Can you work these out from the model? Positions are in its coordinate system, mm. A direction names the side the tool comes from. Give positions to 0.01 mm unless a question says otherwise; leave off trailing zeros. Write each loop counter-clockwise with the first axis right and the second up, starting at its lowest first coordinate (ties: lowest second). Pieces come first, ordered by that corner, then holes.
Autodesk Inventor part; units mm, degrees
ref_plane "YZ Plane" through (0, 0, 0) normal (1, 0, 0) x (0, 1, 0)
ref_plane "XZ Plane" through (0, 0, 0) normal (0, 1, 0) x (-1, 0, 0)
ref_plane "XY Plane" through (0, 0, 0) normal (0, 0, 1) x (1, 0, 0)
sketch "Sketch1" plane through (0, 0, 0) normal (0, 0, 1) x (1, 0, 0)
  line L0 (5, 0) -> (95, 0)
  line L1 (100, 5) -> (100, 26.714)
  line L2 (95, 31.714) -> (5, 31.714)
  line L3 (0, 26.714) -> (0, 5)
  arc A0 (5, 31.714) -> (0, 26.714) centre (5, 26.714) ccw
  arc A1 (0, 5) -> (5, 0) centre (5, 5) ccw
  circle A2 centre (5, 5) radius 2.75
  circle A3 centre (5, 26.714) radius 2.75
  circle A4 centre (25, 26.714) radius 2.75
  circle A5 centre (25, 5) radius 2.75
  arc A6 (100, 26.714) -> (95, 31.714) centre (95, 26.714) ccw
  arc A7 (95, 0) -> (100, 5) centre (95, 5) ccw
  line L4 (125, 20.857) -> (70, 20.857)
  line L5 (70, 20.857) -> (70, 10.857)
  line L6 (70, 10.857) -> (125, 10.857)
  line L7 (130, 15.857) -> (130, 15.857)
  line L8 (130, 20.857) -> (70, 10.857) construction
  line L9 (70, 20.857) -> (130, 10.857) construction
  circle A8 centre (125, 15.857) radius 2.75
  arc A9 (130, 15.857) -> (125, 20.857) centre (125, 15.857) ccw
  arc A10 (125, 10.857) -> (130, 15.857) centre (125, 15.857) ccw
  point P0 (0, 0)
  point P1 (100, 31.714)
  point P2 (100, 0)
  point P3 (100, 15.857)
  point P4 (0, 15.857)
  point P5 (100, 10.857)
  point P6 (100, 20.857)
  dimension "d0" = 100
  dimension "d1" = 31.714
  dimension "d2" = 5
  dimension "d3" = 5.5
  dimension "d4" = 5.5
  dimension "d5" = 21.714
  dimension "d8" = 20
  dimension "d13" = 5
  dimension "d14" = 10
  dimension "d15" = 60
  dimension "d16" = 5.5
  dimension "d17" = 5
  dimension "d18" = 5
extrude "Extrusion1" add sketch "Sketch1" along normal blind 5
properties part number "Arm2"
1) Please list where these lines run through material, in increasing order: L1, parallel to X at y = 27, z = 2.95; L2, parallel to Y at x = 5, z = 3; L3, parallel to Y at x = 125, z = 2.9.
Values follow:
L1: x = 0.01 to 2.26, 7.74 to 22.26, 27.74 to 99.99
L2: y = 0 to 2.25, 7.75 to 23.96, 29.46 to 31.71
L3: y = 10.86 to 13.11, 18.61 to 20.86
2) For pin 1 Ø3 at (y, z) = (25.5, 2.5) entering from +X; pin 2 Ø2.5 at (x, z) = (106.5, 3) entering from -Y, each with a flat end and sliding along its axis, tell me the tip position at first contact or that it passes through.
Values follow:
pin 1: stops at x = 100
pin 2: stops at y = 10.86
3) Suppose I cut it at D-D on y = 9. Write out the boundary of the cut face in (x, z).
Values follow:
outline: (0, 0) - (100, 0) - (100, 5) - (0, 5) - close
4) Suppose I cut it at B-B on z = 2.4. Write out the boundary of the cut face in (x, y).
Values follow:
outline: (0, 5) arc R5 ccw to (5, 0) - (95, 0) arc R5 ccw to (100, 5) - (100, 10.86) - (125, 10.86) arc R5 ccw to (125, 20.86) - (100, 20.86) - (100, 26.71) arc R5 ccw to (95, 31.71) - (5, 31.71) arc R5 ccw to (0, 26.71) - close; hole circle Ø5.5 at (5, 5); hole circle Ø5.5 at (5, 26.71); hole circle Ø5.5 at (25, 5); hole circle Ø5.5 at (25, 26.71); hole circle Ø5.5 at (125, 15.86)
5) For faces 1 (the face through (113, 20.857, 2)), 2 (the face through (100, 8, 2)), 3 (the face through (49, 0, 2)), which set-ups out of +Z, -Z, +X, -X, +Y, -Y let a thin tool reach every point of the face, with its end or its side?
Values follow:
face 1: +Z, -Z, +X, +Y
face 2: +Z, -Z, +X, -Y
face 3: +Z, -Z, +X, -X, -Y
6) Suppose I cut it at A-A on x = 25. Write out the boundary of the cut face in (y, z).
Values follow:
outline: (0, 0) - (2.25, 0) - (2.25, 5) - (0, 5) - close; (7.75, 0) - (23.96, 0) - (23.96, 5) - (7.75, 5) - close; (29.46, 0) - (31.71, 0) - (31.71, 5) - (29.46, 5) - close
7) Suppose I cut it at C-C on y = 14.5. Write out the boundary of the cut face in (x, z).
Values follow:
outline: (0, 0) - (122.61, 0) - (122.61, 5) - (0, 5) - close; (127.39, 0) - (129.81, 0) - (129.81, 5) - (127.39, 5) - close
8) If we mould it in two halves opening along Y, with no side actions, what happens to faces 4 (the face through (1.426, 30.21, 2.465)), 5 (the face through (50, 16, 5)), 6 (the face through (22.253, 4.879, 2.465))? For each: +Y half, -Y half, draft (parallel to the pull), parting line (faces both ways), or undercut.
Values follow:
face 4: +Y half
face 5: draft
face 6: undercut
